from build123d import *

# Parameters (mm, degrees)
F0_R      = 7.9355102155
F1_DEPTH  = 50.8
F2_DEPTH  = 28.575
F3_R      = 7.2928540477
F5_DEPTH  = 5.715
F4_R      = 6.3630946633
F6_DEPTH  = 15.875
F7_R      = 0.4292471714
F8_R      = 4.7645441954
F9_DEPTH  = 15.875
F10_R     = 6.351340122
F11_DEPTH = 50.8


with BuildPart() as f1:
    # F0 (on Top) → F1 (new body)
    with BuildSketch(Plane.XY):
        Circle(F0_R)
    extrude(amount=F1_DEPTH)

    # F2 (add): a face of the model
    f2_faces = [f1.faces().sort_by_distance(p)[0] for p in [
        (0, 0, 0),
    ]]
    extrude(f2_faces, amount=F2_DEPTH)

    # F3 (on face) → F5 (join)
    with BuildSketch(Plane(origin=(0, 0, -28.575), x_dir=(1, 0, 0), z_dir=(0, 0, -1))):
        Circle(F3_R)
    extrude(amount=F5_DEPTH)

    # F4 (on face) → F6 (join)
    with BuildSketch(Plane(origin=(0, 0, -28.575), x_dir=(1, 0, 0), z_dir=(0, 0, -1))):
        Circle(F4_R)
    extrude(amount=F6_DEPTH)

    # F7
    f7_edges = [f1.edges().sort_by_distance(p)[0] for p in [
        (-6.363095, 0, -34.29),
        (-7.292854, 0, -34.29),
    ]]
    fillet(f7_edges, radius=F7_R)

    # F8 (on face) → F9 (cut)
    with BuildSketch(Plane(origin=(0, 0, -44.45), x_dir=(1, 0, 0), z_dir=(0, 0, -1))):
        Circle(F8_R)
    extrude(amount=-F9_DEPTH, mode=Mode.SUBTRACT)

    # F10 (on face) → F11 (cut)
    with BuildSketch(Plane.XY.offset(50.8)):
        Circle(F10_R)
    extrude(amount=-F11_DEPTH, mode=Mode.SUBTRACT)


solid = f1.part
For this review, take the finished solid that the model builds, in its own axes (mm). A direction names the side the tool comes from. Give positions to 0.01 mm unless a question says otherwise; leave off trailing zeros. Order: outer loops, then holes, each group sorted by start corner. A loop starts at its lowest first (then second) coordinate and runs counter-clockwise, first axis right, second up. Notation, with made-up numbers: (-2.5, 42) - (3.5, 42) arc R36 cw to (3.5, 76) - close; hole circle Ø2 at (26, 35.25). An arc over 180 degrees is marked (long way). Answer as a JSON object with one key per item and string values. Group by question number.
Item 1: Take a section at A-A on z = 7. Give the boundary of the cut face in (x, y).
Item 2: Machinability: for faces 1 (the cylindrical face through (-1.38, 6.21, -39.52)), 2 (the flat face through (0, 7, 50.8)), 3 (the cylindrical face through (-1.38, -6.2, 25.76)), which of the approach directions +Z, -Z, +X, -X, +Y, -Y give a long, thin tool a straight path to every point of the face, cutting with its end or side? Answer none if there is none.
Item 3: Draft analysis for pull direction X (two halves, no side actions). For faces 4 (the cylindrical face through (3.365, 6.47, -31.181)), 5 (the flat face through (0, 0, -28.575)), 6 (the flat face through (0, 0, 0)), 7 (the flat face through (-1, -5, -44.45)), state which applies: pulls with the +X half, pulls with the -X half, needs draft (parallel to the pull), parting line crosses it, or undercut.
Item 4: Take a section at D-D on z = -23. Give the boundary of the cut face in (x, y), and give its area (3 significant figures).
Item 5: Clearance check with flat-ended pins moving along their axes: pin 1 Ø8 at (x, z) = (5, -33.5) entering from -Y; pin 2 Ø4 at (x, z) = (5, -1.5) entering from -Y; pin 3 Ø2 at (x, y) = (2, 1.5) entering from -Z (3 decimals). State where each tip first meets the part, or that it passes through.
Item 6: Wall thickness on line 1 along X through (y, z) = (0, -32.25); line 2 along X through (y, z) = (0, -40.5): over which ranges is each line inside the solid? List them lowest first.
Reported:
{
 "1": {"outline": "circle Ø15.87 at (0, 0); hole circle Ø12.7 at (0, 0)"},
 "2": {"face 1": "-Z", "face 2": "+Z, +X, -X, +Y, -Y", "face 3": "+Z"},
 "3": {"face 4": "parting line crosses it", "face 5": "undercut", "face 6": "undercut", "face 7": "needs draft"},
 "4": {"outline": "circle Ø15.87 at (0, 0)", "area": "198 mm^2"},
 "5": {"pin 1": "y = -7.22", "pin 2": "y = -7.35", "pin 3": "z = -28.575"},
 "6": {"line 1": "-7.29 to -4.76, 4.76 to 7.29", "line 2": "-6.36 to -4.76, 4.76 to 6.36"}
}
